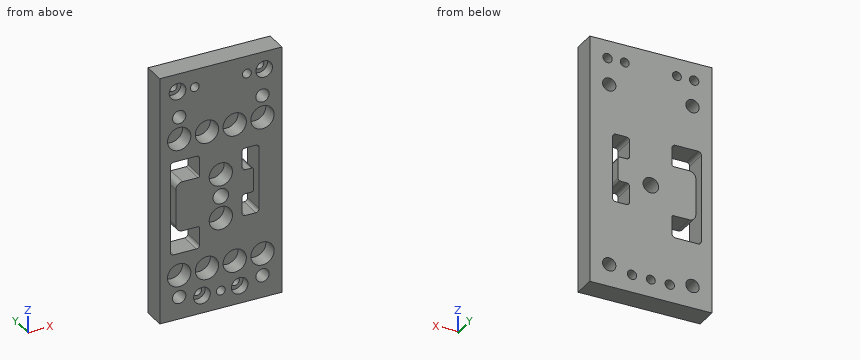
```python
from build123d import *

# Parameters (mm, degrees)
SKETCH1_W                                           = 110
SKETCH1_H                                           = 225
BOSS_EXTRUDE1_DEPTH                                 = 20
CUT_EXTRUDE1_REACH                                  = 128.812
CUT_EXTRUDE2_REACH                                  = 128.812
SKETCH4_R                                           = 10.5
CUT_EXTRUDE3_DEPTH                                  = 14.2
CUT_EXTRUDE4_REACH                                  = 128.812
SKETCH5_R                                           = 6
CUT_EXTRUDE5_REACH                                  = 128.812
SKETCH6_R                                           = 7
CBORE_FOR_M8_HEX_SOCKET_HEAD_CAP_SCREW1_D           = 8.4
CBORE_FOR_M8_HEX_SOCKET_HEAD_CAP_SCREW1_CBORE_D     = 15
CBORE_FOR_M8_HEX_SOCKET_HEAD_CAP_SCREW1_CBORE_DEPTH = 8.6
F_8_0MM_DOWEL_HOLE1_D                               = 8


with BuildPart() as part:
    # Sketch1 → Boss-Extrude1 (new body)
    with BuildSketch(Plane(origin=(0, 0, 0), x_dir=(1, 0, 0), z_dir=(0, 1, 0))):
        Rectangle(SKETCH1_W, SKETCH1_H)
    extrude(amount=BOSS_EXTRUDE1_DEPTH)

    # Sketch2 → Cut-Extrude1 (cut, up to next)
    with BuildSketch(Plane(origin=(0, 20, 0), x_dir=(1, 0, 0), z_dir=(0, 1, 0)), mode=Mode.PRIVATE) as cut_extrude1_sk1:
        with BuildLine():
            Line((-42.5, -32.64), (-22, -32.64))
            ThreePointArc((-22, -32.64), (-19.878679656, -31.761320344), (-19, -29.64))
            Line((-19, -29.64), (-19, -14.14))
            ThreePointArc((-19, -14.14), (-19.439339828, -13.079339828), (-20.5, -12.64))
            Line((-20.5, -12.64), (-34.5, -12.64))
            ThreePointArc((-34.5, -12.64), (-38.742640687, -10.882640687), (-40.5, -6.64))
            Line((-40.5, -6.64), (-40.5, 26.36))
            ThreePointArc((-40.5, 26.36), (-38.742640687, 30.602640687), (-34.5, 32.36))
            Line((-34.5, 32.36), (-20.5, 32.36))
            ThreePointArc((-20.5, 32.36), (-19.439339828, 32.799339828), (-19, 33.86))
            Line((-19, 33.86), (-19, 49.36))
            ThreePointArc((-19, 49.36), (-19.878679656, 51.481320344), (-22, 52.36))
            Line((-22, 52.36), (-42.5, 52.36))
            ThreePointArc((-42.5, 52.36), (-44.621320344, 51.481320344), (-45.5, 49.36))
            Line((-45.5, 49.36), (-45.5, -29.64))
            ThreePointArc((-45.5, -29.64), (-44.621320344, -31.761320344), (-42.5, -32.64))
        make_face()
    cut_extrude1_tool1 = extrude(cut_extrude1_sk1.sketch, amount=-CUT_EXTRUDE1_REACH, mode=Mode.PRIVATE) & part.part
    add(cut_extrude1_tool1.solids().sort_by_distance((-43.991747, 20, -50.851747))[0], mode=Mode.SUBTRACT)

    # Sketch3 → Cut-Extrude2 (cut, up to next)
    with BuildSketch(Plane(origin=(0, 20, 0), x_dir=(1, 0, 0), z_dir=(0, 1, 0)), mode=Mode.PRIVATE) as cut_extrude2_sk1:
        with BuildLine():
            Line((22, -8.64), (27.5, -8.64))
            ThreePointArc((27.5, -8.64), (28.914213562, -8.054213562), (29.5, -6.64))
            Line((29.5, -6.64), (29.5, 11.36))
            ThreePointArc((29.5, 11.36), (28.914213562, 12.774213562), (27.5, 13.36))
            Line((27.5, 13.36), (22, 13.36))
            ThreePointArc((22, 13.36), (19.878679656, 14.238679656), (19, 16.36))
            Line((19, 16.36), (19, 30.36))
            ThreePointArc((19, 30.36), (19.878679656, 32.481320344), (22, 33.36))
            Line((22, 33.36), (31.5, 33.36))
            ThreePointArc((31.5, 33.36), (33.621320344, 32.481320344), (34.5, 30.36))
            Line((34.5, 30.36), (34.5, -25.64))
            ThreePointArc((34.5, -25.64), (33.621320344, -27.761320344), (31.5, -28.64))
            Line((31.5, -28.64), (22, -28.64))
            ThreePointArc((22, -28.64), (19.878679656, -27.761320344), (19, -25.64))
            Line((19, -25.64), (19, -11.64))
            ThreePointArc((19, -11.64), (19.878679656, -9.518679656), (22, -8.64))
        make_face()
    cut_extrude2_tool1 = extrude(cut_extrude2_sk1.sketch, amount=-CUT_EXTRUDE2_REACH, mode=Mode.PRIVATE) & part.part
    add(cut_extrude2_tool1.solids().sort_by_distance((24.75, 20, 9.279081))[0], mode=Mode.SUBTRACT)

    # Sketch4 → Cut-Extrude3 (cut)
    with BuildSketch(Plane.XZ):
        with Locations(Location((37.5, 52.64, 0), (0, 0, 270))):
            Circle(SKETCH4_R)
        with Locations(Location((12.5, 52.64, 0), (0, 0, 270))):
            Circle(SKETCH4_R)
        with Locations(Location((-12.5, 52.64, 0), (0, 0, 270))):
            Circle(SKETCH4_R)
        with Locations(Location((-37.5, 52.64, 0), (0, 0, 270))):
            Circle(SKETCH4_R)
        with Locations(Location((0, 10.14, 0), (0, 0, 270))):
            Circle(SKETCH4_R)
        with Locations(Location((0, -29.86, 0), (0, 0, 270))):
            Circle(SKETCH4_R)
        with Locations(Location((37.5, -72.36, 0), (0, 0, 270))):
            Circle(SKETCH4_R)
        with Locations(Location((12.5, -72.36, 0), (0, 0, 270))):
            Circle(SKETCH4_R)
        with Locations(Location((-12.5, -72.36, 0), (0, 0, 270))):
            Circle(SKETCH4_R)
        with Locations(Location((-37.5, -72.36, 0), (0, 0, 270))):
            Circle(SKETCH4_R)
    extrude(amount=-CUT_EXTRUDE3_DEPTH, mode=Mode.SUBTRACT)

    # Sketch5 → Cut-Extrude4 (cut, up to next)
    with BuildSketch(Plane(origin=(0, 20, 0), x_dir=(1, 0, 0), z_dir=(0, 1, 0)), mode=Mode.PRIVATE) as cut_extrude4_sk1:
        with Locations(Location((-37.5, 92.36, 0), (0, 0, 270))):
            Circle(SKETCH5_R)
    cut_extrude4_tool1 = extrude(cut_extrude4_sk1.sketch, amount=-CUT_EXTRUDE4_REACH, mode=Mode.PRIVATE) & part.part
    # Sketch5 → Cut-Extrude4 (cut, up to next)
    with BuildSketch(Plane(origin=(0, 20, 0), x_dir=(1, 0, 0), z_dir=(0, 1, 0)), mode=Mode.PRIVATE) as cut_extrude4_sk2:
        with Locations(Location((37.5, 92.36, 0), (0, 0, 270))):
            Circle(SKETCH5_R)
    cut_extrude4_tool2 = extrude(cut_extrude4_sk2.sketch, amount=-CUT_EXTRUDE4_REACH, mode=Mode.PRIVATE) & part.part
    # Sketch5 → Cut-Extrude4 (cut, up to next)
    with BuildSketch(Plane(origin=(0, 20, 0), x_dir=(1, 0, 0), z_dir=(0, 1, 0)), mode=Mode.PRIVATE) as cut_extrude4_sk3:
        with Locations(Location((-37.5, -72.64, 0), (0, 0, 270))):
            Circle(SKETCH5_R)
    cut_extrude4_tool3 = extrude(cut_extrude4_sk3.sketch, amount=-CUT_EXTRUDE4_REACH, mode=Mode.PRIVATE) & part.part
    # Sketch5 → Cut-Extrude4 (cut, up to next)
    with BuildSketch(Plane(origin=(0, 20, 0), x_dir=(1, 0, 0), z_dir=(0, 1, 0)), mode=Mode.PRIVATE) as cut_extrude4_sk4:
        with Locations(Location((37.5, -72.64, 0), (0, 0, 270))):
            Circle(SKETCH5_R)
    cut_extrude4_tool4 = extrude(cut_extrude4_sk4.sketch, amount=-CUT_EXTRUDE4_REACH, mode=Mode.PRIVATE) & part.part
    add(cut_extrude4_tool1.solids().sort_by_distance((-37.5, 20, -92.36))[0], mode=Mode.SUBTRACT)
    add(cut_extrude4_tool2.solids().sort_by_distance((37.5, 20, -92.36))[0], mode=Mode.SUBTRACT)
    add(cut_extrude4_tool3.solids().sort_by_distance((-37.5, 20, 72.64))[0], mode=Mode.SUBTRACT)
    add(cut_extrude4_tool4.solids().sort_by_distance((37.5, 20, 72.64))[0], mode=Mode.SUBTRACT)

    # Sketch6 → Cut-Extrude5 (cut, up to next)
    with BuildSketch(Plane(origin=(0, 20, 0), x_dir=(1, 0, 0), z_dir=(0, 1, 0)), mode=Mode.PRIVATE) as cut_extrude5_sk1:
        with Locations(Location((0, 9.86, 0), (0, 0, 270))):
            Circle(SKETCH6_R)
    cut_extrude5_tool1 = extrude(cut_extrude5_sk1.sketch, amount=-CUT_EXTRUDE5_REACH, mode=Mode.PRIVATE) & part.part
    add(cut_extrude5_tool1.solids().sort_by_distance((0, 20, -9.86))[0], mode=Mode.SUBTRACT)

    # CBORE for M8 Hex Socket Head Cap Screw1 (through all)
    with Locations(Plane(origin=(0, 0, 0), x_dir=(-1, 0, 0), z_dir=(0, -1, 0))):
        with Locations((-17, 96.5), (17, 96.5), (-39, -96.5), (39, -96.5)):
            CounterBoreHole(CBORE_FOR_M8_HEX_SOCKET_HEAD_CAP_SCREW1_D / 2, CBORE_FOR_M8_HEX_SOCKET_HEAD_CAP_SCREW1_CBORE_D / 2, CBORE_FOR_M8_HEX_SOCKET_HEAD_CAP_SCREW1_CBORE_DEPTH)

    # Ø8.0mm Dowel Hole1 (through all)
    with Locations(Plane(origin=(0, 0, 0), x_dir=(-1, 0, 0), z_dir=(0, -1, 0))):
        with Locations((0, 96.5), (-23.5, -96.5), (23.5, -96.5)):
            Hole(F_8_0MM_DOWEL_HOLE1_D / 2)


solid = part.part
```
The model under review builds one solid part; all positions refer to its coordinate system, in mm. Round coordinates to 2 decimals unless told otherwise and drop trailing zeros. Loops run counter-clockwise (first coordinate to the right, second up) from the corner with the lowest first, then second, coordinate; pieces in that order, holes last. Notation, with made-up numbers: M -11,55.25 L 0,55.25 A17 ccw 0,80.25 Z; hole C 57,31.25 d5. An arc over 180 degrees is marked long. Answer as a JSON object with one key per item and string values.
(1) Take a section at B-B on z = 52.64. Give the boundary of the cut face in (x, y).
Resolved:
{"outline": "M -55,0 L -48,0 L -48,14.2 L -27,14.2 L -27,0 L -23,0 L -23,14.2 L -2,14.2 L -2,0 L 2,0 L 2,14.2 L 23,14.2 L 23,0 L 27,0 L 27,14.2 L 48,14.2 L 48,0 L 55,0 L 55,20 L -55,20 Z"}
(2) To check wall thickness, follow line 1 along X through (y, z) = (6.75, -72.36); line 2 along X through (y, z) = (7.5, 96.5); line 3 along Z through (x, y) = (12, 14). State the ranges of each line that lie inside material, in increasing order.
Resolved:
{"line 1": "-55 to -48, -27 to -23, -2 to 2, 23 to 27, 48 to 55", "line 2": "-55 to -46.5, -31.5 to -27.5, -19.5 to 19.5, 27.5 to 31.5, 46.5 to 55", "line 3": "-112.5 to -82.85, -61.87 to 42.15, 63.13 to 112.5"}
(3) Take a section at A-A on z = 96.5. Give the boundary of the cut face in (x, y).
Resolved:
{"outline": "M -55,0 L -46.5,0 L -46.5,8.6 L -43.2,8.6 L -43.2,20 L -55,20 Z; M -34.8,8.6 L -31.5,8.6 L -31.5,0 L -27.5,0 L -27.5,20 L -34.8,20 Z; M -19.5,0 L 19.5,0 L 19.5,20 L -19.5,20 Z; M 27.5,0 L 31.5,0 L 31.5,8.6 L 34.8,8.6 L 34.8,20 L 27.5,20 Z; M 43.2,8.6 L 46.5,8.6 L 46.5,0 L 55,0 L 55,20 L 43.2,20 Z"}
(4) Take a section at C-C on y = 11.5. Count the separate pieces of the cut face and the enclosed holes in it, and give its area (3 significant figures).
Resolved:
{"separate pieces": "1", "enclosed holes": "24", "area": "18,300 mm²"}
(5) Clearance check with a flat-ended pin moving along its axis: P1, Ø9.5, axis at x = 37.5, z = -92.36, coming from the -Y side. State where the tip first meets the part, or that it passes through.
Resolved:
{"P1": "through"}
